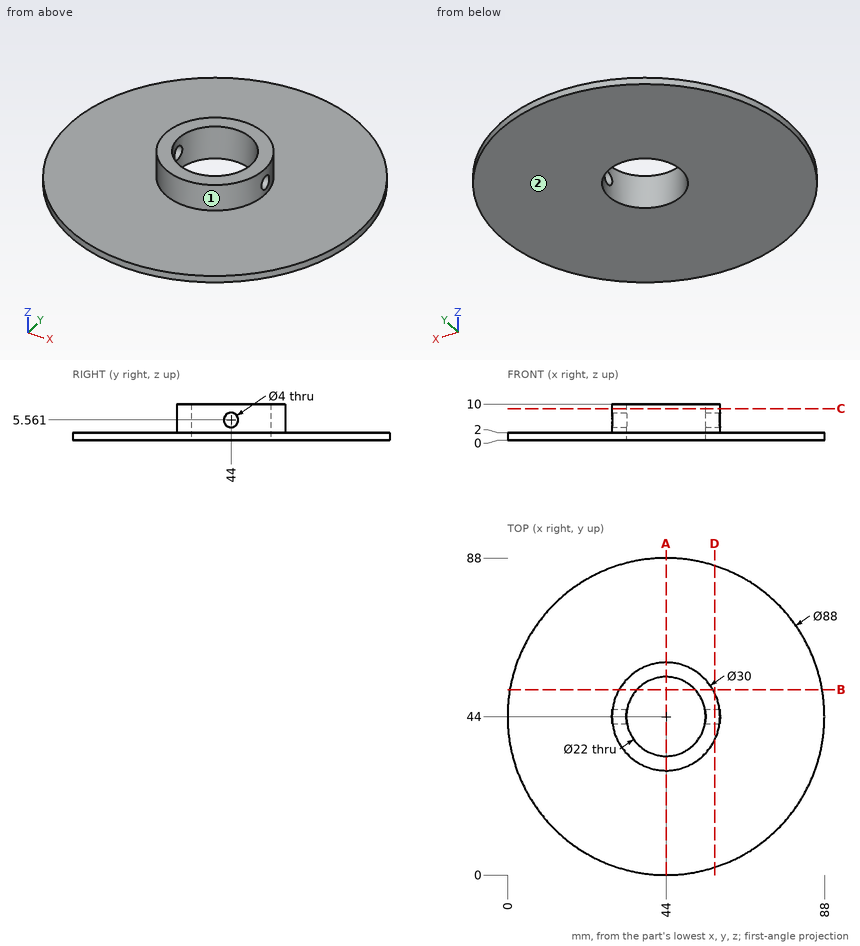
Here's the drawing with two shaded views (mm, measured from the low corner). I have some questions. A direction names the side the tool comes from. Give positions to 0.01 mm unless a question says otherwise; leave off trailing zeros. Loops run counter-clockwise (first coordinate to the right, second up) from the corner with the lowest first, then second, coordinate; pieces in that order, holes last. Notation, with made-up numbers: M 72,47.5 L 80,47.5 A20 cw 80,58.5 Z; hole C 35,63 d8. An arc over 180 degrees is marked long. Use one line per item in the form item = value. Start each with the question number.
(1) I'm going to push flat-ended pins straight in: P1, Ø3.5, axis at y = 44, z = 5.56, coming from the +X side; P2, Ø4, axis at y = 35.5, z = 2, coming from the -X side; P3, Ø2, axis at x = 41, z = 8.5, coming from the +Y side; P4, Ø1, axis at y = 31, z = 7.5, coming from the -X side. Where does each tip first touch, or does it pass through?
(2) Please list where these lines run through material, in increasing order: line 1 (X direction, y = 43.5, z = 9.25); line 2 (Y direction, x = 44, z = 7.75); line 3 (Z direction, x = 57.65, y = 44).
(3) I want a section at C-C, the plane z = 8.75. Write out the boundary of the cut face in (x, y), and give its area (3 significant figures).
(4) I want a section at B-B, the plane y = 51.5. Write out the boundary of the cut face in (x, z).
(5) I want a section at D-D, the plane x = 57.5. Write out the boundary of the cut face in (y, z).
(6) On a 3-axis mill with a long thin cutter (end or side, diameter ignored), from which of +Z, -Z, +X, -X, +Y, -Y can I reach the whole of each face in a straight line? I mean the marked faces 1 and 2. Say none if no direction works.
(7) I want a section at A-A, the plane x = 44. Write out the boundary of the cut face in (y, z), and give its area (3 significant figures).
Worked out:
q1.P1 = through
q1.P2 = 0.48
q1.P3 = 58.87
q1.P4 = 35.71
q2.line_1 = 29.01 to 33.01, 54.99 to 58.99
q2.line_2 = 29 to 33, 55 to 59
q2.line_3 = 0 to 3.56, 7.56 to 10
q3.outline = C 44,44 d30; hole C 44,44 d22
q3.area = 327 mm²
q4.outline = M 0.64,0 L 35.95,0 L 35.95,10 L 31.01,10 L 31.01,2 L 0.64,2 Z; M 52.05,0 L 87.36,0 L 87.36,2 L 56.99,2 L 56.99,10 L 52.05,10 Z
q5.outline = M 2.12,0 L 85.88,0 L 85.88,2 L 50.54,2 L 50.54,10 L 37.46,10 L 37.46,2 L 2.12,2 Z; hole C 44,5.56 d4
q6.face_1 = +Z
q6.face_2 = -Z, +X, -X, +Y, -Y
q7.outline = M 0,0 L 33,0 L 33,10 L 29,10 L 29,2 L 0,2 Z; M 55,0 L 88,0 L 88,2 L 59,2 L 59,10 L 55,10 Z
q7.area = 196 mm²
